Autodesk Inventor part; units mm, degrees
ref_plane "YZ Plane" through (0, 0, 0) normal (1, 0, 0) x (0, 1, 0)
ref_plane "XZ Plane" through (0, 0, 0) normal (0, 1, 0) x (-1, 0, 0)
ref_plane "XY Plane" through (0, 0, 0) normal (0, 0, 1) x (1, 0, 0)
sketch "スケッチ1" plane through (0, 0, 0) normal (0, 0, 1) x (1, 0, 0)
  line L0 (-13.75, -7.5) -> (13.75, -7.5)
  line L1 (13.75, -7.5) -> (13.75, 7.5)
  line L2 (13.75, 7.5) -> (-13.75, 7.5)
  line L3 (-13.75, 7.5) -> (-13.75, -7.5)
  line L4 (-13.75, -7.5) -> (13.75, 7.5) construction
  line L5 (13.75, -7.5) -> (-13.75, 7.5) construction
  point P0 (0, 0)
  dimension "d0" = 27.5
  dimension "d1" = 15
extrude "押し出し1" add sketch "スケッチ1" along normal blind 75
sketch "スケッチ2" plane through (0, 0, 75) normal (0, 0, 1) x (1, 0, 0)
  line L0 (-13.75, 5) -> (13.75, 5)
  line L1 (13.75, 5) -> (13.75, -5)
  line L2 (13.75, -5) -> (-13.75, -5)
  line L3 (-13.75, -5) -> (-13.75, 5)
  line L4 (-13.75, 5) -> (13.75, -5) construction
  line L5 (13.75, 5) -> (-13.75, -5) construction
  point P0 (0, 0)
  dimension "d4" = 27.5
  dimension "d5" = 10
extrude "押し出し2" add sketch "スケッチ2" along normal blind 11
chamfer "面取り1" distance 2 angle 45 2 edges at (0, 7.5, 75) (0, -7.5, 75)
sketch "スケッチ3" plane through (0, 0, 86) normal (0, 0, 1) x (1, 0, 0)
  line L0 (13.75, -5) -> (13.75, 5)
  line L1 (13.75, -5) -> (-13.75, -5)
  line L2 (13.75, 5) -> (-3.25, 5)
  line L3 (-3.25, 5) -> (-3.25, -5)
  line L4 (-3.25, -5) -> (13.75, -5)
  line L5 (13.75, -5) -> (13.75, 5)
  point P0 (0, 0)
  dimension "d11" = 17
extrude "押し出し3" add sketch "スケッチ3" along normal blind 5
sketch "スケッチ4" plane through (0, 0, 91) normal (0, 0, 1) x (1, 0, 0)
  line L0 (3.75, -3.75) -> (10.75, -3.75)
  line L1 (10.75, -3.75) -> (10.75, 3.75)
  line L2 (10.75, 3.75) -> (3.75, 3.75)
  line L3 (3.75, 3.75) -> (3.75, -3.75)
  line L4 (3.75, -3.75) -> (10.75, 3.75) construction
  line L5 (10.75, -3.75) -> (3.75, 3.75) construction
  line L6 (13.75, -5) -> (13.75, 5)
  point P0 (0, 0)
  point P1 (7.25, 0)
  dimension "d14" = 7
  dimension "d15" = 7.5
  dimension "d16" = 3
extrude "押し出し4" add sketch "スケッチ4" along normal blind 8.5
sketch "スケッチ5" plane through (13.75, -7.5, 0) normal (1, 0, 0) x (0, 0, -1)
  line L0 (0, 7.5) -> (-91, 7.5) construction
  line L1 (-91, 2.5) -> (-91, 12.5)
  line L2 (0, 0) -> (0, 15)
  point P0 (-25.5, 7.5)
  point P1 (-40.5, 7.5)
  dimension "d19" = 25.5
  dimension "d20" = 15
hole "穴1" at (13.75, 0, 25.5) at (13.75, 0, 40.5) direction (-1, 0, 0) diameter 10 depth 8 tip angle 118
sketch "スケッチ6" plane through (-13.75, -7.5, 0) normal (-1, 0, 0) x (0, 0, 1)
  line L0 (0, 7.5) -> (86, 7.5) construction
  line L1 (86, 2.5) -> (86, 12.5)
  line L2 (0, 15) -> (0, 0)
  point P0 (34, 7.5)
  point P1 (19, 7.5)
  point P2 (49, 7.5)
  dimension "d28" = 19
  dimension "d29" = 15
  dimension "d30" = 15
hole "穴2" at (-13.75, 0, 34) at (-13.75, 0, 19) at (-13.75, 0, 49) direction (1, 0, 0) diameter 10 depth 8 tip angle 118
sketch "スケッチ7" plane through (-13.75, 7.5, 0) normal (0, 1, 0) x (1, 0, 0)
  line L0 (27.5, 0) -> (0, 0)
  line L1 (5, 0) -> (5, -72.92) construction
  line L2 (0, 0) -> (0, -73)
  point P0 (13.75, 0)
  point P1 (5, -26)
  point P2 (5, -39.5)
  dimension "d38" = 5
  dimension "d39" = 26
  dimension "d40" = 13.5
hole "穴3" at (-8.75, 7.5, 26) at (-8.75, 7.5, 39.5) direction (0, -1, 0) diameter 3 depth 8 tip angle 118
sketch "スケッチ8" plane through (13.75, -7.5, 0) normal (1, 0, 0) x (0, 0, -1)
  line L0 (0, 7.5) -> (-99.5, 7.5) construction
  line L1 (-99.5, 3.75) -> (-99.5, 11.25)
  circle A0 centre (-62, 7.5) radius 2.75
  line L2 (0, 0) -> (0, 15)
  dimension "d48" = 5.5
  dimension "d49" = 62
extrude "押し出し5" add sketch "スケッチ8" along normal blind 4
properties part number "solenoid _valve_sa"
Source: CAD feature listing. Evaluate the final solid. Frame: model axes, mm. A direction names the side the tool comes from. Coordinates: 2 decimals unless noted, no trailing zeros. Loops run counter-clockwise (first coordinate to the right, second up) from the corner with the lowest first, then second, coordinate; pieces in that order, holes last. Notation, with made-up numbers: (60, 82) - (104, 82) arc R10 ccw to (104, 97) - close; hole circle Ø3 at (36.5, 33). An arc over 180 degrees is marked (long way). One line per item, written item: value. Start each with the question number.
1. Contact query for flat-ended pins moving along their axis: P1, Ø8, axis at y = 0, z = 34, coming from the +X side; P2, Ø1.5, axis at y = 0, z = 88, coming from the -X side; P3, Ø5.5, axis at x = 6.5, z = 96.5, coming from the -Y side. Output: stop coordinate, or through.
2. Mould query, pull axis X, two halves, no side actions, for faces 4 (the conical face through (-8.85, -1.245, 26.241)), 5 (the flat face through (-13.75, 0, 42)), 6 (the flat face through (0, -5, 83)). Classes: pulls with the +X half, pulls with the -X half, needs draft (parallel to the pull), parting line crosses it, or undercut.
3. Section C-C (z = 78). Return the cut outline in (x, y), and give its area (3 significant figures).
4. Ray query, L1, parallel to Z at x = 12, y = 0; L2, parallel to Z at x = 8, y = 0; L3, parallel to Z at x = -7, y = 0.25. Return the intervals inside material, ascending.
5. Set-up query: faces 1 (the flat face through (-9, 0, 86)), 2 (the cylindrical face through (9.694, -0.22, 30.495)), 3 (the cylindrical face through (-10, 0, 29)). Return all of +Z, -Z, +X, -X, +Y, -Y with unobstructed straight access to the full face (end or side cutting, diameter ignored); none if empty.
6. Section B-B (x = 1.5). Return the cut outline in (y, z), and give its area (3 significant figures).
7. Section A-A (z = 62). Return the cut outline in (x, y), and give its area (4 significant figures).
Verdict:
1. P1: stops at x = 13.75
1. P2: stops at x = -3.25
1. P3: stops at y = -3.75
2. face 4: undercut
2. face 5: pulls with the -X half
2. face 6: needs draft
3. outline: (-13.75, -5) - (13.75, -5) - (13.75, 5) - (-13.75, 5) - close
3. area: 275 mm2
4. L1: z = 0 to 20.5, 30.5 to 35.5, 45.5 to 91
4. L2: z = 0 to 20.5, 30.5 to 35.5, 45.5 to 99.5
4. L3: z = 0 to 14.01, 23.99 to 29.01, 38.99 to 44.01, 53.99 to 86
5. face 1: +Z, -X, +Y, -Y
5. face 2: +X
5. face 3: -X
6. outline: (-7.5, 0) - (7.5, 0) - (7.5, 73) - (5.5, 75) - (5, 75) - (5, 91) - (-5, 91) - (-5, 75) - (-5.5, 75) - (-7.5, 73) - close
6. area: 1,280 mm2
7. outline: (-13.75, -7.5) - (13.75, -7.5) - (13.75, -2.75) - (17.75, -2.75) - (17.75, 2.75) - (13.75, 2.75) - (13.75, 7.5) - (-13.75, 7.5) - close
7. area: 434.5 mm2
